Input: part model. Units: mm. Frame: model coordinates. A direction names the side the tool comes from. Round coordinates to 2 decimals unless told otherwise and drop trailing zeros. Order: outer loops, then holes, each group sorted by start corner. A loop starts at its lowest first (then second) coordinate and runs counter-clockwise, first axis right, second up. Notation, with made-up numbers: (-35, -34.75) -> (-18, -34.75) arc R14 ccw to (-18, -23.75) -> close; hole circle Ø8 at (26, -9). An arc over 180 degrees is marked (long way). Answer as CSV lines item,"result". Start each with the question number.
1) First-contact query: P1, Ø1, axis at x = 426, y = -397.5, coming from the -Z side. Flat tip, straight axial feed; report the tip coordinate or a pass-through.
2) Access query for faces 4 (the face through (975, -950, -746)), 5 (the face through (-950, -975, -746)), 6 (the face through (950, -494, -1025)). Directions: +Z, -Z, +X, -X, +Y, -Y. A direction counts if a zero-diameter tool reaches every point of the face in a straight line with its end or side. Return the directions, or none.
3) Mould query, pull axis Z, two halves, no side actions, for faces 1 (the face through (-14, 0, 80)), 2 (the face through (950, -975, -746)), 3 (the face through (-14, -493, 500)). Classes: +Z half, -Z half, draft (parallel to the pull), parting line (faces both ways), or undercut.
4) Section query B-B, the plane z = -640.5. Output: boundary loops of the cut face in (x, y), and give its area (3 significant figures).
5) Line query: L1, parallel to Z at x = 881, y = -919.5. Output: solid intervals per line, ascending.
6) Section query C-C, the plane y = -738. Output: boundary loops of the cut face in (x, z), and give its area (4 significant figures).
7) Section query A-A, the plane x = 693.5. Output: boundary loops of the cut face in (y, z).
```python
from build123d import *

# Parameters (mm, degrees)
F0_W     = 2000
F0_H     = 1000
F1_DEPTH = 1000
F3_W     = 50
F3_H     = 50
F4_DEPTH = 500
F6_W     = 2000
F6_H     = 1000
F6_W_2   = 1900
F6_H_2   = 900
F7_DEPTH = 50


with BuildPart() as f1:
    # F0 (on Front) → F1 (new body)
    with BuildSketch(Plane.XZ):
        Rectangle(F0_W, F0_H)
    extrude(amount=F1_DEPTH)

    # F3 (on offset) → F4 (join)
    with BuildSketch(Plane(origin=(0, 0, -500), x_dir=(1, 0, 0), z_dir=(0, 0, -1))):
        with Locations((975, 25)):
            Rectangle(F3_W, F3_H)
        with Locations((975, 975)):
            Rectangle(F3_W, F3_H)
        with Locations((-975, 975)):
            Rectangle(F3_W, F3_H)
        with Locations((-975, 25)):
            Rectangle(F3_W, F3_H)
    extrude(amount=F4_DEPTH)

    # F6 (on offset) → F7 (join)
    with BuildSketch(Plane(origin=(0, 0, -1000), x_dir=(1, 0, 0), z_dir=(0, 0, -1))):
        with Locations((0, 500)):
            Rectangle(F6_W, F6_H)
        with Locations((0, 500)):
            Rectangle(F6_W_2, F6_H_2, mode=Mode.SUBTRACT)
    extrude(amount=F7_DEPTH)


solid = f1.part
```
Findings:
1,P1,"stops at z = -500"
2,face 4,"+X, -X"
2,face 5,"+Y, -Y"
2,face 6,"-Z"
3,face 1,"draft"
3,face 2,"undercut"
3,face 3,"+Z half"
4,outline,"(-1000, -1000) -> (-950, -1000) -> (-950, -950) -> (-1000, -950) -> close; (-1000, -50) -> (-950, -50) -> (-950, 0) -> (-1000, 0) -> close; (950, -1000) -> (1000, -1000) -> (1000, -950) -> (950, -950) -> close; (950, -50) -> (1000, -50) -> (1000, 0) -> (950, 0) -> close"
4,area,"10,000 mm^2"
5,L1,"z = -500 to 500"
6,outline,"(-1000, -1050) -> (-950, -1050) -> (-950, -1000) -> (-1000, -1000) -> close; (-1000, -500) -> (1000, -500) -> (1000, 500) -> (-1000, 500) -> close; (950, -1050) -> (1000, -1050) -> (1000, -1000) -> (950, -1000) -> close"
6,area,"2,005,000 mm^2"
7,outline,"(-1000, -1050) -> (-950, -1050) -> (-950, -1000) -> (-1000, -1000) -> close; (-1000, -500) -> (0, -500) -> (0, 500) -> (-1000, 500) -> close; (-50, -1050) -> (0, -1050) -> (0, -1000) -> (-50, -1000) -> close"
